Part model, mm, in its own coordinate system. A direction names the side the tool comes from. Give positions to 0.01 mm unless a question says otherwise; leave off trailing zeros. Order: outer loops, then holes, each group sorted by start corner. A loop starts at its lowest first (then second) coordinate and runs counter-clockwise, first axis right, second up.
1. Probe line 1 (Y direction, x = 3.5, z = 5.55); line 2 (Z direction, x = 2.75, y = -1.5); line 3 (Y direction, x = 0, z = 35). List the from-to ranges inside material, lowest first.
2. Mould opens along Y. For faces 6 (the cylindrical face through (0.108, -0.488, -1.521)), 7 (the flat face through (1.95, 2.23, 5.51)), 8 (the cylindrical face through (2.31, 0.38, 5.51)) say: +Y half, -Y half, draft (parallel to the pull), parting line (faces both ways), or undercut.
3. Which spindle directions (+Z, -Z, +X, -X, +Y, -Y) get a long thin tool onto all of the face, cutting with end or side? Do faces 1 (the cylindrical face through (0.065, 3.535, -3.504)), 2 (the flat face through (2, 1, 6)), 3 (the flat face through (0, 0, 40)), 4 (the flat face through (1, 0, 0)), 5 (the flat face through (1.9, -2.24, 5.51)). Say none if no direction does.
4. Slice it at B-B on z = 26. List the corners of the cut face in (x, y), and give its area (3 significant figures).
5. Slice it at C-C on y = 4.25. List the corners of the cut face in (x, z).
6. Slice it at A-A on x = 4.25. List the corners of the cut face in (y, z).
7. Drop flat-ended pins along their axis: pin 1 Ø1.5 at (x, y) = (3.5, 0) entering from +Z; pin 2 Ø2 at (x, y) = (4.5, -0.5) entering from +Z; pin 3 Ø1.5 at (x, y) = (0, 0) entering from -Z; pin 4 Ø1 at (x, y) = (0, -0.5) entering from -Z. Give the stop position or say it passes through.
8. Slice it at D-D on x = 1.25. List the corners of the cut face in (y, z).
from build123d import *

# Parameters (mm, degrees)
SKETCH1_R           = 1.75
BOSS_EXTRUDE1_DEPTH = 40
SKETCH16_R          = 1.25
BOSS_EXTRUDE2_DEPTH = 1
SWEEP1_PROFILE_R    = 0.5


with BuildPart() as part:
    # Sketch1 → Boss-Extrude1 (new body)
    with BuildSketch(Plane.XY):
        Circle(SKETCH1_R)
    extrude(amount=BOSS_EXTRUDE1_DEPTH)

    # Sketch16 → Boss-Extrude2 (add)
    with BuildSketch(Plane(origin=(0, 0, 6), x_dir=(-1, 0, 0), z_dir=(0, 0, -1))):
        with BuildLine():
            Line((-3.851561771, 1.968858634), (0, 2.5))
            ThreePointArc((0, 2.5), (2.5, 0), (0, -2.5))
            Line((0, -2.5), (-3.851561771, -1.968858634))
            ThreePointArc((-3.851561771, -1.968858634), (-5.5, 0), (-3.851561771, 1.968858634))
        make_face()
        with Locations((-3.5, 0)):
            Circle(SKETCH16_R, mode=Mode.SUBTRACT)
    extrude(amount=BOSS_EXTRUDE2_DEPTH)

    # Sweep1: sweep along a curve in space
    with BuildLine() as sweep1_path:
        Line((0, 0, 0), (0, 0, -3))
        ThreePointArc((0, 0, -3), (0, 0.292893219, -3.707106781), (0, 1, -4))
        Line((0, 1, -4), (0, 6, -4))
    # Sweep1 profile (on start of the path) → Sweep1 (sweep)
    with BuildSketch(Plane(origin=(0, 0, 0), x_dir=(-1, 0, 0), z_dir=(0, 0, -1))):
        Circle(SWEEP1_PROFILE_R)
    sweep(path=sweep1_path.line)


solid = part.part
Data:
1. line 1: y = -2.02 to -1.25, 1.25 to 2.02
1. line 2: z = 5 to 6
1. line 3: y = -1.75 to 1.75
2. face 6: parting line
2. face 7: +Y half
2. face 8: undercut
3. face 1: +Y
3. face 2: +Z
3. face 3: +Z, +X, -X, +Y, -Y
3. face 4: none
3. face 5: +Z, -Z, +X, -Y
4. outline: circle Ø3.5 at (0, 0)
4. area: 9.62 mm2
5. outline: circle Ø1 at (0, -4)
6. outline: (-1.85, 5) - (-1, 5) - (-1, 6) - (-1.85, 6) - close; (1, 5) - (1.85, 5) - (1.85, 6) - (1, 6) - close
7. pin 1: passes through
7. pin 2: stops at z = 6
7. pin 3: stops at z = -4.48
7. pin 4: stops at z = -4.12
8. outline: (-2.33, 5) - (-1.22, 5) - (-1.22, 0) - (1.22, 0) - (1.22, 5) - (2.33, 5) - (2.33, 6) - (1.22, 6) - (1.22, 40) - (-1.22, 40) - (-1.22, 6) - (-2.33, 6) - close
